Read the model definition and answer for the solid it produces. Units are mm, in the model's axes. A direction names the side the tool comes from. Round coordinates to 2 decimals unless told otherwise and drop trailing zeros. Order: outer loops, then holes, each group sorted by start corner. A loop starts at its lowest first (then second) coordinate and runs counter-clockwise, first axis right, second up. Notation, with made-up numbers: (-36, 59.5) - (13, 59.5) arc R23 ccw to (13, 67.5) - close; hole circle Ø10 at (-24.5, 40). An arc over 180 degrees is marked (long way). Answer as a JSON object with one key per item and string values. Group by question number.
Q1. The mould has two halves that part along X. Classify faces 1 (the flat face through (-5, -46.666, -207)), 2 (the flat face through (9, -29, -338.609)), 3 (the flat face through (-44.45, -19, 87)): pulls with the +X half, pulls with the -X half, needs draft (parallel to the pull), parting line crosses it, or undercut.
Q2. A cutting plane is placed at A-A on y = -35.5. Determine the outline of the cut face in (x, z), and give its area (3 significant figures).
Q3. A cutting plane is placed at C-C on y = 0.5. Determine the outline of the cut face in (x, z).
Q4. A cutting plane is placed at B-B on x = -26.5. Determine the outline of the cut face in (y, z), and give its area (3 significant figures).
Q5. Consider line 1 (Z direction, x = 35, y = -43.5); line 2 (Z direction, x = 0, y = 6); line 3 (Z direction, x = 0, y = -53.5). Determine where each line is inside the solid, lowest interval first.
Q6. A tool of negligible diameter and unlimited length cuts with its end or side. For faces 4 (the flat face through (-19, -24.441, -306)), 5 (the flat face through (6.35, 1, 500)), 6 (the cylindrical face through (-14.041, -54.714, -198.734)), from which of +Z, -Z, +X, -X, +Y, -Y can it reach the whole face along a straight path? Write none if from no direction.
Q7. Given pin 1 Ø15 at (x, z) = (-6.5, 502.5) entering from -Y; pin 2 Ø10 at (x, z) = (0, -211.61) entering from -Y; pin 3 Ø15 at (y, z) = (-5, -300.5) entering from +X; pin 4 Ø11.5 at (x, z) = (-2.5, -217.5) entering from -Y, each flat-ended and moving along its own axis, determine where each tip first touches the part or whether it passes through.
```python
from build123d import *

# Parameters (mm, degrees)
F1_DEPTH      = 44.45
F2_R          = 5.08
F4_DEPTH      = 50.8
F5_R          = 6.35
F6_DEPTH      = 26.360464475
F6_DEPTH_BACK = 62.541535525
F7_R          = 19.05
F7_R_2        = 6.35
F8_DEPTH      = 15.875


with BuildPart() as f1:
    # F0 (on Right) → F1 (new body, symmetric)
    with BuildSketch(Plane.YZ):
        Polygon((26.359464475, -364.0086964671), (26.359464475, 524.9913035329), (-24.440535525, 524.9913035329), (-24.440535525, 474.1913035329), (-62.540535525, 474.1913035329), (-62.540535525, -275.1086964671), (-24.440535525, -275.1086964671), (-24.440535525, -338.6086964671), (-62.540535525, -338.6086964671), (-62.540535525, -364.0086964671), align=None)
    extrude(amount=F1_DEPTH, both=True)

    # F2
    f2_edges = [f1.edges().sort_by_distance(p)[0] for p in [
        (44.45, -62.540536, 99.541304),
        (44.45, -62.540536, -351.308696),
        (-44.45, -62.540536, -351.308696),
        (-44.45, -62.540536, 99.541304),
        (44.45, 26.359464, 80.491304),
        (-44.45, 26.359464, 80.491304),
    ]]
    fillet(f2_edges, radius=F2_R)

    # F3 (on Front) → F4 (cut, symmetric)
    with BuildSketch(Plane.XZ):
        Polygon((44.45, 474.1913035329), (44.45, 524.9913035329), (6.35, 524.9913035329), (6.35, 474.1913035329), (39.37, 474.1913035329), align=None)
        Polygon((44.45, -275.1086964671), (39.37, -275.1086964671), (6.35, -275.1086964671), (6.35, -338.6086964671), (39.37, -338.6086964671), (44.45, -338.6086964671), align=None)
    extrude(amount=F4_DEPTH, both=True, mode=Mode.SUBTRACT)

    # F5 (on Front) → F6 (cut, two sides)
    with BuildSketch(Plane.XZ) as f6_sk:
        with Locations((0, -211.6086964671)):
            Circle(F5_R)
    extrude(amount=-F6_DEPTH, mode=Mode.SUBTRACT)
    extrude(f6_sk.sketch, amount=F6_DEPTH_BACK, mode=Mode.SUBTRACT)

    # F7 (on face) → F8 (cut)
    with BuildSketch(Plane.XZ.offset(62.540535525)):
        with Locations((0, -211.6086964671)):
            Circle(F7_R)
        with Locations((0, -211.6086964671)):
            Circle(F7_R_2, mode=Mode.SUBTRACT)
    extrude(amount=-F8_DEPTH, mode=Mode.SUBTRACT)


solid = f1.part
```
Result set:
{
 "1": {"face 1": "undercut", "face 2": "needs draft", "face 3": "pulls with the -X half"},
 "2": {"outline": "(-44.45, -364.01) - (44.45, -364.01) - (44.45, -338.61) - (-44.45, -338.61) - close; (-44.45, -275.11) - (44.45, -275.11) - (44.45, 474.19) - (-44.45, 474.19) - close; hole circle Ø12.7 at (0, -211.61)", "area": "68,700 mm²"},
 "3": {"outline": "(-44.45, -364.01) - (44.45, -364.01) - (44.45, -338.61) - (6.35, -338.61) - (6.35, -275.11) - (44.45, -275.11) - (44.45, 474.19) - (6.35, 474.19) - (6.35, 524.99) - (-44.45, 524.99) - close; hole circle Ø12.7 at (0, -211.61)"},
 "4": {"outline": "(-62.54, -364.01) - (26.36, -364.01) - (26.36, 524.99) - (-24.44, 524.99) - (-24.44, 474.19) - (-62.54, 474.19) - (-62.54, -275.11) - (-24.44, -275.11) - (-24.44, -338.61) - (-62.54, -338.61) - close", "area": "74,700 mm²"},
 "5": {"line 1": "z = -364.01 to -338.61, -275.11 to 474.19", "line 2": "z = -364.01 to -217.96, -205.26 to 524.99", "line 3": "z = -364.01 to -338.61, -275.11 to -230.66, -192.56 to 474.19"},
 "6": {"face 4": "+X, -X, -Y", "face 5": "+Z, +X, +Y, -Y", "face 6": "-Y"},
 "7": {"pin 1": "stops at y = -24.44", "pin 2": "passes through", "pin 3": "stops at x = 6.35", "pin 4": "stops at y = -46.67"}
}
